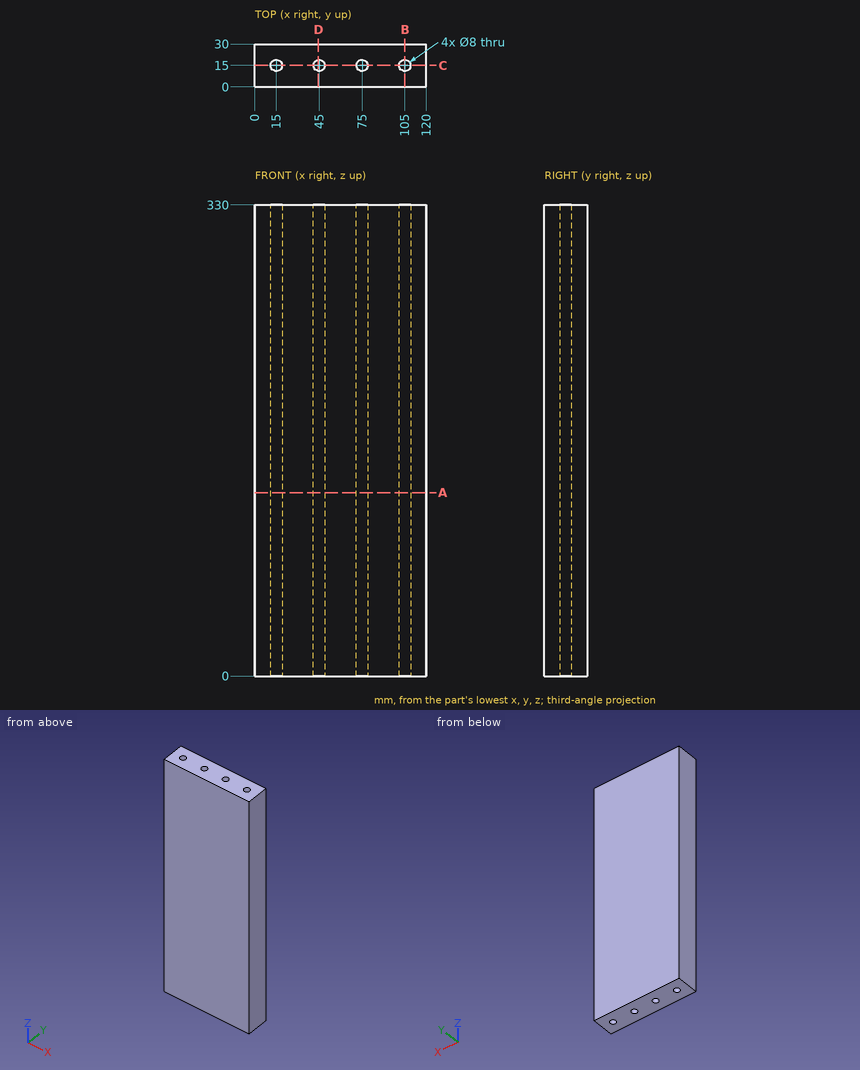
Here's the drawing with two shaded views (mm, measured from the low corner). I have some questions. Give positions to 0.01 mm unless a question says otherwise; leave off trailing zeros. Order: outer loops, then holes, each group sorted by start corner. A loop starts at its lowest first (then second) coordinate and runs counter-clockwise, first axis right, second up. Notation, with made-up numbers: (-6.5, 16) - (14.5, 16) arc R15 ccw to (14.5, 38) - close; hole circle Ø5 at (-1.75, 19). An arc over 180 degrees is marked (long way). Use a Markdown table: item, result. Add a question column.
Q1. If we section it at A-A on z = 128.5: Write out the boundary of the cut face in (x, y), plus the area to 3 significant figures.
Q2. Please list where these lines run through material, in increasing order: line 1 along X through (y, z) = (14, 253); line 2 along Y through (x, z) = (75, 187); line 3 along X through (y, z) = (11.5, 193.5).
Q3. If we section it at C-C on y = 15: Write out the boundary of the cut face in (x, z), plus the area to 3 significant figures.
Q4. If we section it at D-D on x = 44.5: Write out the boundary of the cut face in (y, z), plus the area to 3 significant figures.
Q5. If we section it at B-B on x = 105: Write out the boundary of the cut face in (y, z), plus the area to 3 significant figures.
Answers follow:
| question | item | result |
|---|---|---|
| 1 | outline | (0, 0) - (120, 0) - (120, 30) - (0, 30) - close; hole circle Ø8 at (15, 15); hole circle Ø8 at (45, 15); hole circle Ø8 at (75, 15); hole circle Ø8 at (105, 15) |
| 1 | area | 3,400 mm^2 |
| 2 | line 1 | x = 0 to 11.13, 18.87 to 41.13, 48.87 to 71.13, 78.87 to 101.13, 108.87 to 120 |
| 2 | line 2 | y = 0 to 11, 19 to 30 |
| 2 | line 3 | x = 0 to 13.06, 16.94 to 43.06, 46.94 to 73.06, 76.94 to 103.06, 106.94 to 120 |
| 3 | outline | (0, 0) - (11, 0) - (11, 330) - (0, 330) - close; (19, 0) - (41, 0) - (41, 330) - (19, 330) - close; (49, 0) - (71, 0) - (71, 330) - (49, 330) - close; (79, 0) - (101, 0) - (101, 330) - (79, 330) - close; (109, 0) - (120, 0) - (120, 330) - (109, 330) - close |
| 3 | area | 29,000 mm^2 |
| 4 | outline | (0, 0) - (11.03, 0) - (11.03, 330) - (0, 330) - close; (18.97, 0) - (30, 0) - (30, 330) - (18.97, 330) - close |
| 4 | area | 7,280 mm^2 |
| 5 | outline | (0, 0) - (11, 0) - (11, 330) - (0, 330) - close; (19, 0) - (30, 0) - (30, 330) - (19, 330) - close |
| 5 | area | 7,260 mm^2 |
